```python
from build123d import *

# Parameters (mm, degrees)
BOSS_EXTRUDE1_DEPTH = 5.842


with BuildPart() as part:
    # Sketch1 → Boss-Extrude1 (new body)
    with BuildSketch(Plane.XY):
        Polygon((-38, 18.796), (-63.6, 18.796), (-63.6, 12.954), (-74.4474, 12.954), (-74.4474, 9.779), (-73.152, 9.779), (-73.152, 6.604), (-74.4474, 6.604), (-74.4474, 5.896), (-77.9526, 5.896), (-77.9526, 6.604), (-79.248, 6.604), (-79.248, 9.779), (-77.9526, 9.779), (-77.9526, 12.954), (-88.8, 12.954), (-88.8, 18.796), (-114.4, 18.796), (-114.4, 12.954), (-117.475, 12.954), (-117.475, -12.954), (-114.4, -12.954), (-114.4, -18.796), (-88.8, -18.796), (-88.8, -12.954), (-77.9526, -12.954), (-77.9526, -9.779), (-79.248, -9.779), (-79.248, -6.604), (-77.9526, -6.604), (-77.9526, -5.896), (-74.4474, -5.896), (-74.4474, -6.604), (-73.152, -6.604), (-73.152, -9.779), (-74.4474, -9.779), (-74.4474, -12.954), (-63.6, -12.954), (-63.6, -18.796), (-38, -18.796), (-38, -12.954), (-27.1526, -12.954), (-27.1526, -9.779), (-28.448, -9.779), (-28.448, -6.604), (-27.1526, -6.604), (-27.1526, -5.896), (-23.6474, -5.896), (-23.6474, -6.604), (-22.352, -6.604), (-22.352, -9.779), (-23.6474, -9.779), (-23.6474, -12.954), (-12.8, -12.954), (-12.8, -18.796), (12.8, -18.796), (12.8, -12.954), (23.6474, -12.954), (23.6474, -9.779), (22.352, -9.779), (22.352, -6.604), (23.6474, -6.604), (23.6474, -5.896), (27.1526, -5.896), (27.1526, -6.604), (28.448, -6.604), (28.448, -9.779), (27.1526, -9.779), (27.1526, -12.954), (38, -12.954), (38, -18.796), (63.6, -18.796), (63.6, -12.954), (74.4474, -12.954), (74.4474, -9.779), (73.152, -9.779), (73.152, -6.604), (74.4474, -6.604), (74.4474, -5.896), (77.9526, -5.896), (77.9526, -6.604), (79.248, -6.604), (79.248, -9.779), (77.9526, -9.779), (77.9526, -12.954), (88.8, -12.954), (88.8, -18.796), (114.4, -18.796), (114.4, -12.954), (117.475, -12.954), (117.475, 12.954), (114.4, 12.954), (114.4, 18.796), (88.8, 18.796), (88.8, 12.954), (77.9526, 12.954), (77.9526, 9.779), (79.248, 9.779), (79.248, 6.604), (77.9526, 6.604), (77.9526, 5.896), (74.4474, 5.896), (74.4474, 6.604), (73.152, 6.604), (73.152, 9.779), (74.4474, 9.779), (74.4474, 12.954), (63.6, 12.954), (63.6, 18.796), (38, 18.796), (38, 12.954), (27.1526, 12.954), (27.1526, 9.779), (28.448, 9.779), (28.448, 6.604), (27.1526, 6.604), (27.1526, 5.896), (23.6474, 5.896), (23.6474, 6.604), (22.352, 6.604), (22.352, 9.779), (23.6474, 9.779), (23.6474, 12.954), (12.8, 12.954), (12.8, 18.796), (-12.8, 18.796), (-12.8, 12.954), (-23.6474, 12.954), (-23.6474, 9.779), (-22.352, 9.779), (-22.352, 6.604), (-23.6474, 6.604), (-23.6474, 5.896), (-27.1526, 5.896), (-27.1526, 6.604), (-28.448, 6.604), (-28.448, 9.779), (-27.1526, 9.779), (-27.1526, 12.954), (-38, 12.954), align=None)
    extrude(amount=BOSS_EXTRUDE1_DEPTH)


solid = part.part
```
For this review, take the finished solid that the model builds, in its own axes (mm). A direction names the side the tool comes from. Coordinates: 2 decimals unless noted, no trailing zeros. Order: outer loops, then holes, each group sorted by start corner. A loop starts at its lowest first (then second) coordinate and runs counter-clockwise, first axis right, second up. Notation, with made-up numbers: (28.25, 39.5) -> (37.25, 39.5) arc R21 cw to (37.25, 75.5) -> close; hole circle Ø9 at (79, 8). An arc over 180 degrees is marked (long way). Use CSV: the item, a comma, the result in double quotes. Start each with the question number.
Item 1: For faces 4 (the face through (69, 12.954, 3)), 5 (the face through (38, -16, 3)), 6 (the face through (114.4, 16, 3)), 7 (the face through (-51, 18.796, 3)), list the 3-axis set-ups (+Z, -Z, +X, -X, +Y, -Y) from which the entire face can be reached by the end or side of a thin tool; tool diameter is ignored.
Item 2: Insertion check: pin 1 (0.6 mm diameter, centred on x = -74, z = 4.5, fed in from +Y); pin 2 (2.5 mm diameter, centred on x = 116, z = 2.5, fed in from -Y); pin 3 (3 mm diameter, centred on y = -15.5, z = 3, fed in from -X). Each pin has a flat end and moves straight along its axis. Give the tip position at first contact, or say it passes through.
Item 3: Wall thickness on probe 1 along X at (y, z) = (-13.5, 0.5); probe 2 along X at (y, z) = (9.5, 4.7) (3 decimals); probe 3 along Y at (x, z) = (-88, 3.4): over which ranges is each line inside the solid? List them lowest first.
Item 4: Draft analysis for pull direction X (two halves, no side actions). For faces 1 (the face through (12.8, -16, 3)), 2 (the face through (102, 18.796, 3)), 3 (the face through (-114.4, 16, 3)), state which applies: pulls with the +X half, pulls with the -X half, needs draft (parallel to the pull), parting line crosses it, or undercut.
Item 5: We need section A-A, the plane x = 34. Give the boundary of the cut face in (y, z), then the cut area to 3 significant figures.
Derived:
1,face 4,"+Z, -Z, +Y"
1,face 5,"+Z, -Z, -Y"
1,face 6,"+Z, -Z, +X, +Y"
1,face 7,"+Z, -Z, +X, -X, +Y"
2,pin 1,"stops at y = 12.95"
2,pin 2,"stops at y = -12.95"
2,pin 3,"stops at x = -114.4"
3,probe 1,"x = -114.4 to -88.8, -63.6 to -38, -12.8 to 12.8, 38 to 63.6, 88.8 to 114.4"
3,probe 2,"x = -117.475 to -79.248, -73.152 to -28.448, -22.352 to 22.352, 28.448 to 73.152, 79.248 to 117.475"
3,probe 3,"y = -12.95 to 12.95"
4,face 1,"undercut"
4,face 2,"needs draft"
4,face 3,"pulls with the -X half"
5,outline,"(-12.95, 0) -> (12.95, 0) -> (12.95, 5.84) -> (-12.95, 5.84) -> close"
5,area,"151 mm^2"
